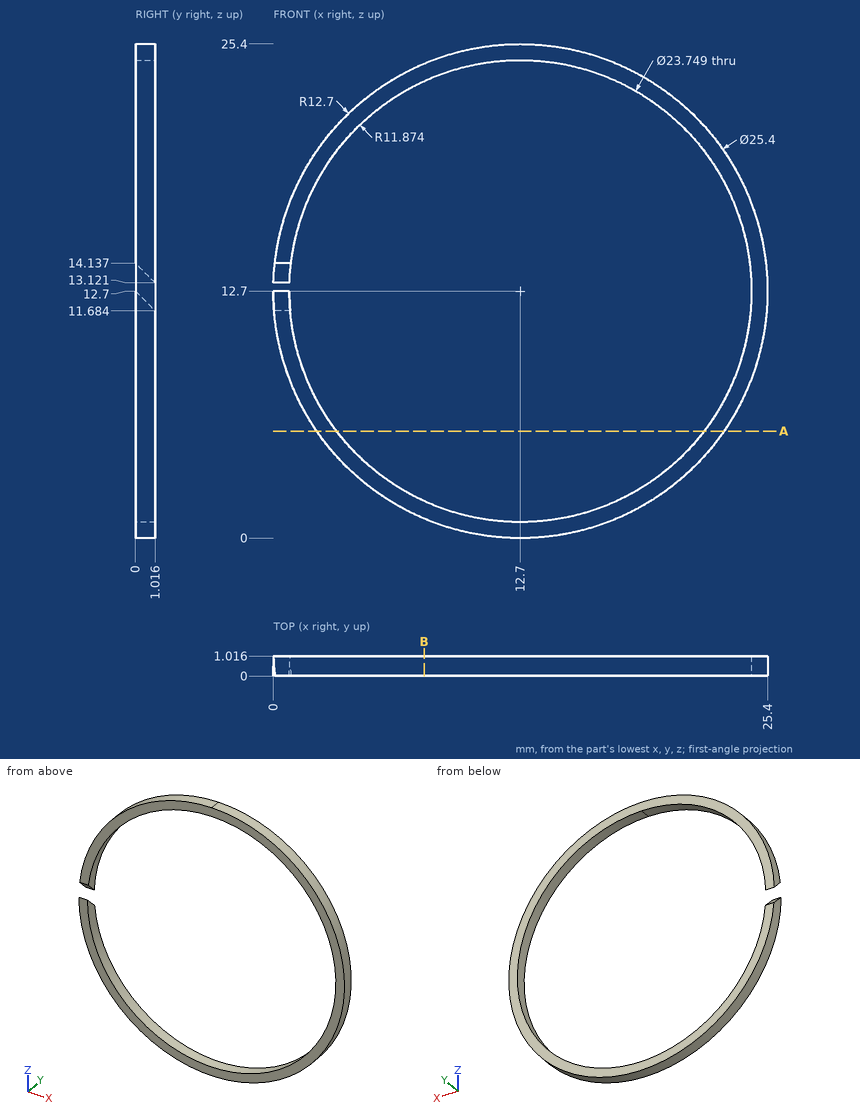
Source: three-view drawing plus pictorial views. Frame: mm from the lowest corner of the part. Give positions to 0.01 mm unless a question says otherwise; leave off trailing zeros. Order: outer loops, then holes, each group sorted by start corner. A loop starts at its lowest first (then second) coordinate and runs counter-clockwise, first axis right, second up. Notation, with made-up numbers: (-31, 57.5) -> (-12, 57.5) arc R21 cw to (-12, 89.5) -> close; hole circle Ø2 at (33, 31.25). An arc over 180 degrees is marked (long way). Write each question's results on one line, items separated by ' | '. Start each with the question number.
Item 1: Cut plane B-B on x = 7.75. Return the cut outline in (y, z) (1 decimal).
Item 2: Cut plane A-A on z = 5.5. Return the cut outline in (x, y) (1 decimal).
Item 3: Line query: line 1 (Z direction, x = 12.7, y = 0.35) (1 decimal); line 2 (X direction, y = 0.7, z = 12.7) (1 decimal); line 3 (Z direction, x = 3.5, y = 0.4) (1 decimal). Output: solid intervals per line, ascending.
Established:
1) outline: (0, 1) -> (1, 1) -> (1, 1.9) -> (0, 1.9) -> close; (0, 23.5) -> (1, 23.5) -> (1, 24.4) -> (0, 24.4) -> close
2) outline: (2.2, 0) -> (3.3, 0) -> (3.3, 1) -> (2.2, 1) -> close; (22.1, 0) -> (23.2, 0) -> (23.2, 1) -> (22.1, 1) -> close
3) line 1: 0 to 0.8, 24.6 to 25.4 | line 2: 24.6 to 25.4 | line 3: 3.9 to 5.2, 20.2 to 21.5
